The model under review builds one solid part; all positions refer to its coordinate system, in mm. Face numbers are marked on the shaded views. A direction names the side the tool comes from. Coordinates: 2 decimals unless noted, no trailing zeros. Loops run counter-clockwise (first coordinate to the right, second up) from the corner with the lowest first, then second, coordinate; pieces in that order, holes last. Notation, with made-up numbers: M -7,1.25 L 47,1.25 A30 ccw 47,29.25 Z; hole C -7,-34.75 d10. An arc over 180 degrees is marked long. Use CSV: the item, a comma, the result in double quotes. Start each with the question number.
1. Clearance check with a flat-ended pin moving along its axis: P1, Ø1.5, axis at x = 0, y = -2.5, coming from the -Z side (3 decimals). State where the tip first meets the part, or that it passes through.
2. Add section A-A, the plane y = -8. Write out the cut boundary in (x, z) (3 decimals), then the cut area to 3 significant figures.
3. For L1, parallel to Z at x = 0.1, y = -6; L2, parallel to Y at x = 0.9, z = -0.55; L3, parallel to Z at x = 0.35, y = -10, list the stretches that pass through material, from the lowest coordinate up.
4. Tool access review of the marked faces 1 and 2: name each direction out of +Z, -Z, +X, -X, +Y, -Y from which nothing blocks a thin tool from reaching the whole face with its end or side.
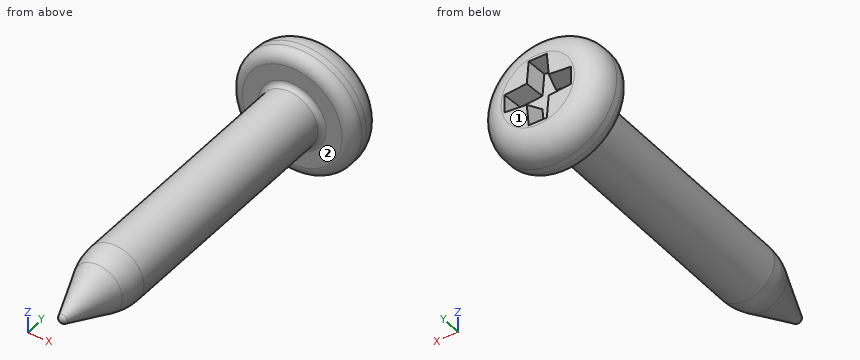
from build123d import *

# Parameters (mm, degrees)
CUT_EXTRUDE1_DEPTH = 0.5
CUT_EXTRUDE1_TAPER = 15


with BuildPart() as part:
    # Sketch1 → Revolve1 (revolve)
    with BuildSketch(Plane.XY):
        with BuildLine():
            Line((0.875, -8.964405423), (0.875, -1.45))
            ThreePointArc((0.875, -1.45), (0.918933983, -1.343933983), (1.025, -1.3))
            Line((1.025, -1.3), (1.5, -1.3))
            ThreePointArc((1.5, -1.3), (1.747487373, -1.197487373), (1.85, -0.95))
            Line((1.85, -0.95), (1.85, -0.75))
            ThreePointArc((1.85, -0.75), (1.630330086, -0.219669914), (1.1, 0))
            Line((1.1, 0), (0, 0))
            Line((0, 0), (0, -11.3))
            ThreePointArc((0, -11.3), (0.084334338, -11.274047247), (0.139485899, -11.205169593))
            Line((0.139485899, -11.205169593), (0.734811985, -9.7))
            ThreePointArc((0.734811985, -9.7), (0.839640421, -9.338822324), (0.875, -8.964405423))
        make_face()
    revolve(axis=Axis((0, 0, 0), (0, -1, 0)))

    # Sketch2 → Cut-Extrude1 (cut)
    with BuildSketch(Plane(origin=(0, 0, 0), x_dir=(1, 0, 0), z_dir=(0, 1, 0))):
        Polygon((-0.271382595, 1), (-0.33, 0.33), (-1, 0.271382595), (-1, -0.271382595), (-0.33, -0.33), (-0.271382595, -1), (0.271382595, -1), (0.33, -0.33), (1, -0.271382595), (1, 0.271382595), (0.33, 0.33), (0.271382595, 1), align=None)
    extrude(amount=-CUT_EXTRUDE1_DEPTH, taper=CUT_EXTRUDE1_TAPER, mode=Mode.SUBTRACT)


solid = part.part
Computed:
1,P1,"stops at z = -0.875"
2,outline,"C 0,0 d1.75"
2,area,"2.41 mm^2"
3,L1,"z = -0.87 to 0.87"
3,L2,"y = -1.3 to 0"
3,L3,"z = -0.51 to 0.51"
4,face 1,"+Z, -Z, +X, -X, +Y"
4,face 2,"-Y"
